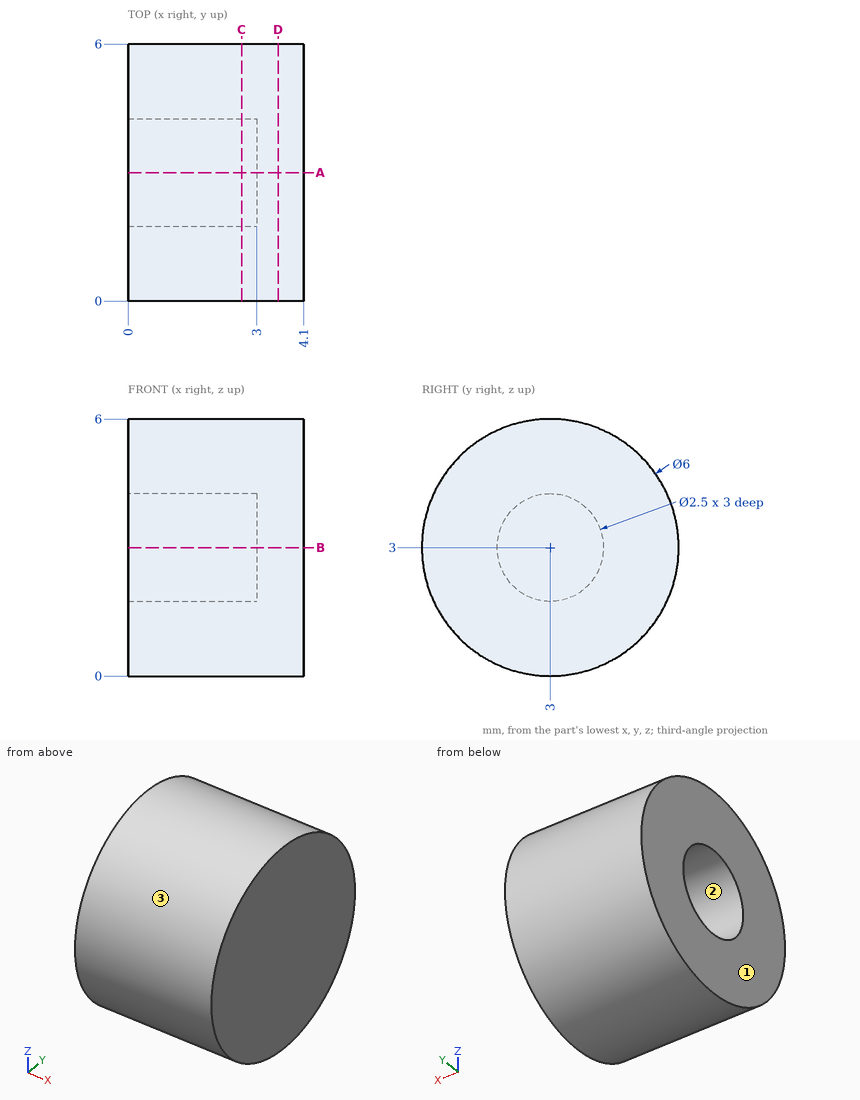
Design review of the part shown in the three views and the two pictorial views. Dimensions are in mm from the part's minimum x, y and z. Give positions to 0.01 mm unless a question says otherwise; leave off trailing zeros. Write each loop counter-clockwise with the first axis right and the second up, starting at its lowest first coordinate (ties: lowest second). Pieces come first, ordered by that corner, then holes. Notation, with made-up numbers: M -5,-5 L 54,-5 A22 ccw 54,10 Z; hole C 58,89 d5. An arc over 180 degrees is marked long. Answer as CSV lines item,"result".
1. Consider section D-D, the plane x = 3.5. Write out the cut boundary in (y, z).
Findings:
outline,"C 3,3 d6"
2. Consider section C-C, the plane x = 2.65. Write out the cut boundary in (y, z).
Findings:
outline,"C 3,3 d6; hole C 3,3 d2.5"
3. For pin 1 (1.2 mm diameter, centred on y = 3, z = 2.5, fed in from -X); pin 2 (1 mm diameter, centred on x = 2, y = 2, fed in from +Z); pin 3 (1 mm diameter, centred on x = 1.5, z = 1, fed in from -Y), all flat-tipped, find the tip position at first contact; note any pin that passes through.
Findings:
pin 1,"stops at x = 3"
pin 2,"stops at z = 5.96"
pin 3,"stops at y = 0.4"
4. Draft analysis for pull direction Z (two halves, no side actions). For the marked faces 1, 2 and 3, state which applies: +Z half, -Z half, draft (parallel to the pull), parting line (faces both ways), or undercut.
Findings:
face 1,"draft"
face 2,"undercut"
face 3,"parting line"
5. Wall thickness on line 1 (Y direction, x = 0.3, z = 3.05); line 2 (X direction, y = 2.95, z = 3.85); line 3 (Z direction, x = 2.25, y = 2.75): over which ranges is each line inside the solid? List them lowest first.
Findings:
line 1,"y = 0 to 1.75, 4.25 to 6"
line 2,"x = 3 to 4.1"
line 3,"z = 0.01 to 1.78, 4.22 to 5.99"
6. Consider section A-A, the plane y = 3. Write out the cut boundary in (x, z).
Findings:
outline,"M 0,0 L 4.1,0 L 4.1,6 L 0,6 L 0,4.25 L 3,4.25 L 3,1.75 L 0,1.75 Z"
